from build123d import *

# Parameters (mm, degrees)
SZKIC1_W                    = 14
SZKIC1_H                    = 25
DODANIE_WYCI_GNI_CIE1_DEPTH = 5
SZKIC2_W                    = 4
SZKIC2_H                    = 19
WYTNIJ_WYCI_GNI_CIE1_DEPTH  = 5
ZAOKR_GLENIE1_R             = 2
ZAOKR_GLENIE2_R             = 3
SZKIC3_R                    = 7
SZKIC3_R_2                  = 3.05
DODANIE_WYCI_GNI_CIE2_DEPTH = 30
DODANIE_WYCI_GNI_CIE3_DEPTH = 5
SZKIC5_R                    = 5
SZKIC5_R_2                  = 2.2
DODANIE_WYCI_GNI_CIE4_DEPTH = 1
SZKIC6_R                    = 3.6
WYTNIJ_WYCI_GNI_CIE2_DEPTH  = 22


with BuildPart() as part:
    # Szkic1 → Dodanie-wyciągnięcie1 (new body)
    with BuildSketch(Plane.XY):
        with Locations((7, 12.5)):
            Rectangle(SZKIC1_W, SZKIC1_H)
    extrude(amount=DODANIE_WYCI_GNI_CIE1_DEPTH)

    # Szkic2 → Wytnij-wyciągnięcie1 (cut)
    with BuildSketch(Plane.XY.offset(5)):
        with Locations((7, 12.5)):
            Rectangle(SZKIC2_W, SZKIC2_H)
    extrude(amount=-WYTNIJ_WYCI_GNI_CIE1_DEPTH, mode=Mode.SUBTRACT)

    # Zaokrąglenie1
    zaokr_glenie1_edges = [part.edges().sort_by_distance(p)[0] for p in [
        (5, 3, 2.5),
        (9, 3, 2.5),
        (9, 22, 2.5),
        (5, 22, 2.5),
    ]]
    fillet(zaokr_glenie1_edges, radius=ZAOKR_GLENIE1_R - 0.0001)  # a hair under: the kernel refuses the full size

    # Zaokrąglenie2
    zaokr_glenie2_edges = [part.edges().sort_by_distance(p)[0] for p in [
        (14, 0, 2.5),
        (0, 0, 2.5),
    ]]
    fillet(zaokr_glenie2_edges, radius=ZAOKR_GLENIE2_R)

    # Szkic3 → Dodanie-wyciągnięcie2 (add)
    with BuildSketch(Plane.XY):
        with Locations(Location((7, 30, 0), (0, 0, 225.584691403))):
            Circle(SZKIC3_R)
        with Locations((7, 30)):
            Circle(SZKIC3_R_2, mode=Mode.SUBTRACT)
    extrude(amount=DODANIE_WYCI_GNI_CIE2_DEPTH)

    # Szkic4 → Dodanie-wyciągnięcie3 (add)
    with BuildSketch(Plane(origin=(0, 0, 0), x_dir=(-1, 0, 0), z_dir=(0, 0, -1))):
        Polygon((-14, 25), (-14, 30), (-11.004847048, 25), align=None)
        Polygon((-2.101020514, 25), (0, 30), (0, 25), align=None)
    extrude(amount=-DODANIE_WYCI_GNI_CIE3_DEPTH)

    # Szkic5 → Dodanie-wyciągnięcie4 (add)
    with BuildSketch(Plane(origin=(0, 0, 0), x_dir=(-1, 0, 0), z_dir=(0, 0, -1))):
        with Locations((-7, 30)):
            Circle(SZKIC5_R)
        with Locations((-7, 30)):
            Circle(SZKIC5_R_2, mode=Mode.SUBTRACT)
    extrude(amount=-DODANIE_WYCI_GNI_CIE4_DEPTH)

    # Szkic6 → Wytnij-wyciągnięcie2 (cut)
    with BuildSketch(Plane.XY.offset(30)):
        with Locations((7, 30)):
            Circle(SZKIC6_R)
    extrude(amount=-WYTNIJ_WYCI_GNI_CIE2_DEPTH, mode=Mode.SUBTRACT)


solid = part.part
Geometry: final body of the model. Coordinates: model frame, mm. A direction names the side the tool comes from. Coordinates: 2 decimals unless noted, no trailing zeros. Order: outer loops, then holes, each group sorted by start corner. A loop starts at its lowest first (then second) coordinate and runs counter-clockwise, first axis right, second up.
1) First-contact query: P1, Ø3, axis at y = 33, z = 7, coming from the -X side; P2, Ø5, axis at x = 8.5, y = 28.5, coming from the +Z side; P3, Ø2, axis at x = 2, z = 13, coming from the +Y side; P4, Ø1.5, axis at x = 12.5, z = 7.5, coming from the +Y side. Flat tips, straight axial feed; report the tip coordinate or a pass-through.
Result sheet:
P1: stops at x = 0.16
P2: stops at z = 30
P3: stops at y = 35.74
P4: stops at y = 35.14
2) Section D-D (y = 4). Return loops of the section in (x, z), then the cut area to 3 significant figures.
Result sheet:
outline: (0, 0) - (5.27, 0) - (5.27, 5) - (0, 5) - close; (8.73, 0) - (14, 0) - (14, 5) - (8.73, 5) - close
area: 52.7 mm2
3) Section B-B (x = 6.5). Return loops of the section in (y, z), then the cut area to 3 significant figures.
Result sheet:
outline: (0, 0) - (3.06, 0) - (3.06, 5) - (0, 5) - close; (21.94, 0) - (27.86, 0) - (27.86, 1) - (26.99, 1) - (26.99, 8) - (26.43, 8) - (26.43, 30) - (23.02, 30) - (23.02, 5) - (21.94, 5) - close; (32.14, 0) - (36.98, 0) - (36.98, 30) - (33.57, 30) - (33.57, 8) - (33.01, 8) - (33.01, 1) - (32.14, 1) - close
area: 236 mm2
4) Section A-A (y = 10.5). Return loops of the section in (x, z), then the cut area to 3 significant figures.
Result sheet:
outline: (0, 0) - (5, 0) - (5, 5) - (0, 5) - close; (9, 0) - (14, 0) - (14, 5) - (9, 5) - close
area: 50.0 mm2
5) Section C-C (x = 1). Return loops of the section in (y, z), then the cut area to 3 significant figures.
Result sheet:
outline: (0.76, 0) - (33.61, 0) - (33.61, 30) - (26.39, 30) - (26.39, 5) - (0.76, 5) - close
area: 344 mm2
6) Ray query, probe 1 along Y at (x, z) = (7, 4.25); probe 2 along Y at (x, z) = (7, 6.5); probe 3 along Y at (x, z) = (7, 21.75). Return the intervals inside material, ascending.
Result sheet:
probe 1: y = 0 to 3, 22 to 26.95, 33.05 to 37
probe 2: y = 23 to 26.95, 33.05 to 37
probe 3: y = 23 to 26.4, 33.6 to 37
7) Set-up query: faces 4 (the cylindrical face through (5.6, 21.43, 2.46)), 5 (the cylindrical face through (6.339, 27.023, 4.451)), 6 (the cylindrical face through (13.1, 0.86, 2.54)). Return all of +Z, -Z, +X, -X, +Y, -Y with unobstructed straight access to the full face (end or side cutting, diameter ignored); none if empty.
Result sheet:
face 4: +Z, -Z
face 5: +Z
face 6: +Z, -Z, +X, -Y
8) Draft query along X for faces 1 (the cylindrical face through (0.86, 0.9, 2.54)), 2 (the flat face through (4, 12, 5)), 3 (the flat face through (5, 32, 1)). Return one class per face: released by +X, released by -X, zero draft, split by the parting line, or undercut.
Result sheet:
face 1: released by -X
face 2: zero draft
face 3: undercut
